Could you check a few things on this drawing? It's one solid part, dimensions in mm from its lowest x, y, z. A direction names the side the tool comes from. Round coordinates to 2 decimals unless told otherwise and drop trailing zeros. Write each loop counter-clockwise with the first axis right and the second up, starting at its lowest first coordinate (ties: lowest second). Pieces come first, ordered by that corner, then holes. Notation, with made-up numbers: (6.25, 0.5) -> (26.25, 0.5) arc R16 ccw to (26.25, 27.5) -> close; hole circle Ø2 at (-7.75, -8). An arc over 180 degrees is marked (long way). Answer in a Markdown table with one row per item.
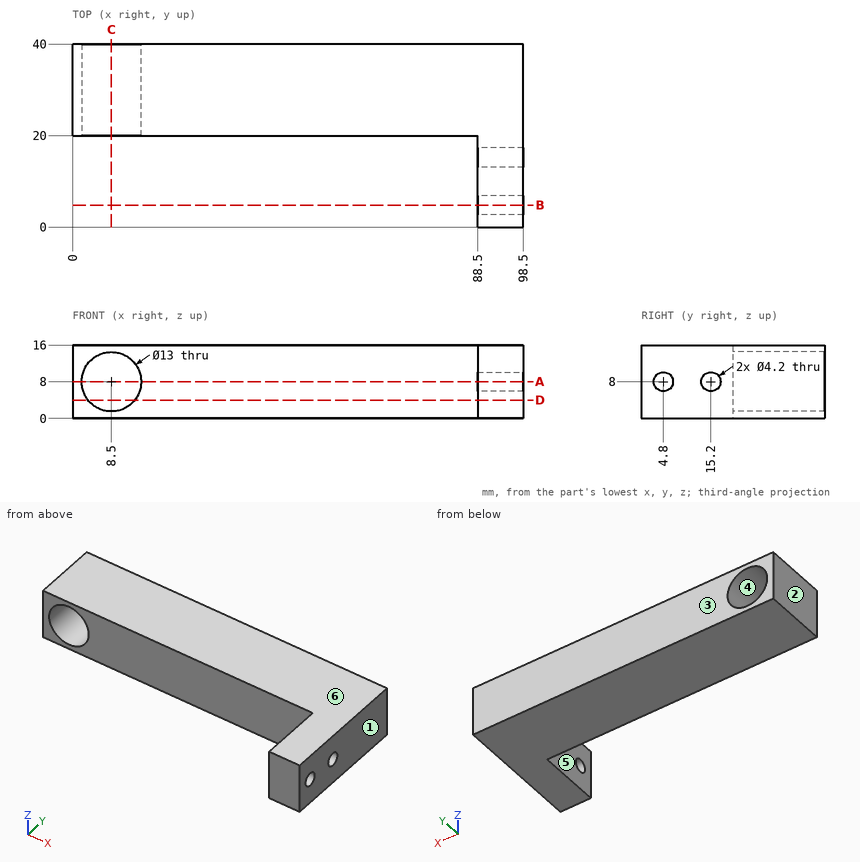
1) For pin 1 (6.5 mm diameter, centred on y = 4.8, z = 8, fed in from -X); pin 2 (6 mm diameter, centred on x = 12.5, y = 14.5, fed in from -Z); pin 3 (4 mm diameter, centred on x = 63.5, y = 19.5, fed in from -Z); pin 4 (2 mm diameter, centred on x = 56.5, z = 8.5, fed in from -Y), each with a flat end and sliding along its axis, tell me the tip position at first contact or that it passes through.
Findings:
| item | result |
|---|---|
| pin 1 | stops at x = 88.5 |
| pin 2 | passes through |
| pin 3 | stops at z = 0 |
| pin 4 | stops at y = 20 |
2) Imagine slicing it at D-D, the plane z = 4. Please give me the cut outline in (x, y).
Findings:
| item | result |
|---|---|
| outline | (0, 20) -> (3.38, 20) -> (3.38, 40) -> (0, 40) -> close; (13.62, 20) -> (88.5, 20) -> (88.5, 0) -> (98.5, 0) -> (98.5, 40) -> (13.62, 40) -> close |
3) Imagine slicing it at A-A, the plane z = 8. Please give me the cut outline in (x, y).
Findings:
| item | result |
|---|---|
| outline | (0, 20) -> (2, 20) -> (2, 40) -> (0, 40) -> close; (15, 20) -> (88.5, 20) -> (88.5, 17.3) -> (98.5, 17.3) -> (98.5, 40) -> (15, 40) -> close; (88.5, 0) -> (98.5, 0) -> (98.5, 2.7) -> (88.5, 2.7) -> close; (88.5, 6.9) -> (98.5, 6.9) -> (98.5, 13.1) -> (88.5, 13.1) -> close |
4) Imagine slicing it at B-B, the plane y = 4.8. Please give me the cut outline in (x, z).
Findings:
| item | result |
|---|---|
| outline | (88.5, 0) -> (98.5, 0) -> (98.5, 5.9) -> (88.5, 5.9) -> close; (88.5, 10.1) -> (98.5, 10.1) -> (98.5, 16) -> (88.5, 16) -> close |
5) Imagine slicing it at C-C, the plane x = 8.5. Please give me the cut outline in (y, z).
Findings:
| item | result |
|---|---|
| outline | (20, 0) -> (40, 0) -> (40, 1.5) -> (20, 1.5) -> close; (20, 14.5) -> (40, 14.5) -> (40, 16) -> (20, 16) -> close |
6) For the marked faces 5 and 6, which set-ups out of +Z, -Z, +X, -X, +Y, -Y let a thin tool reach every point of the face, with its end or its side?
Findings:
| item | result |
|---|---|
| face 5 | +Z, -Z, -X, -Y |
| face 6 | +Z, +X, -X, +Y, -Y |
7) Please list where these lines run through material, in increasing order: line 1 (Y direction, x = 92.5, z = 8); line 2 (X direction, y = 30, z = 8); line 3 (Y direction, x = 59, z = 12.5).
Findings:
| item | result |
|---|---|
| line 1 | y = 0 to 2.7, 6.9 to 13.1, 17.3 to 40 |
| line 2 | x = 0 to 2, 15 to 98.5 |
| line 3 | y = 20 to 40 |
8) Thinking about a two-plate mould opening in X: for the marked faces 1, 2, 3 and 4, which applies, +X half, -X half, draft (parallel to the pull), parting line (faces both ways), or undercut?
Findings:
| item | result |
|---|---|
| face 1 | +X half |
| face 2 | -X half |
| face 3 | draft |
| face 4 | undercut |
